Verification items for the finished model (mm, model axes). Face numbers are marked on the shaded views. A direction names the side the tool comes from. Coordinates: 2 decimals unless noted, no trailing zeros. Order: outer loops, then holes, each group sorted by start corner. A loop starts at its lowest first (then second) coordinate and runs counter-clockwise, first axis right, second up. Notation, with made-up numbers: (-22, 88) -> (-14, 88) arc R24 cw to (-14, 120) -> close; hole circle Ø4 at (4.25, 1.5). An arc over 180 degrees is marked (long way). Answer as CSV lines item,"result".
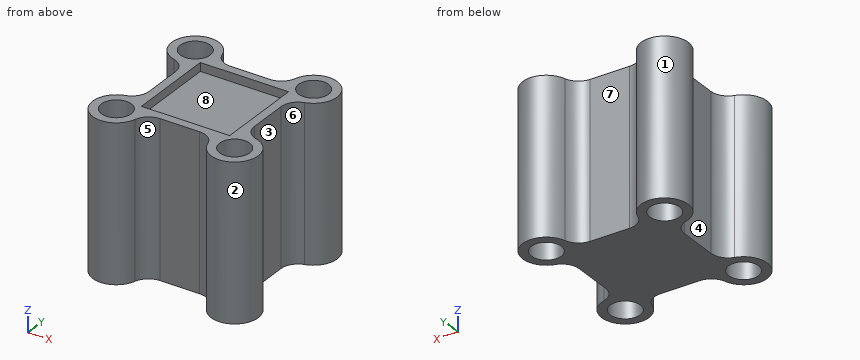
Autodesk Inventor part; units mm, degrees
ref_plane "YZ Plane" through (0, 0, 0) normal (1, 0, 0) x (0, 1, 0)
ref_plane "XZ Plane" through (0, 0, 0) normal (0, 1, 0) x (-1, 0, 0)
ref_plane "XY Plane" through (0, 0, 0) normal (0, 0, 1) x (1, 0, 0)
sketch "Sketch1" plane through (0, 0, 0) normal (0, 0, 1) x (1, 0, 0)
  line L0 (6.15, -6.15) -> (-6.15, -6.15)
  line L1 (-6.15, -6.15) -> (-6.15, 6.15)
  line L2 (-6.15, 6.15) -> (6.15, 6.15)
  line L3 (6.15, 6.15) -> (6.15, -6.15)
  line L4 (6.15, -6.15) -> (-6.15, 6.15) construction
  line L5 (-6.15, -6.15) -> (6.15, 6.15) construction
  line L6 (5.15, -5.15) -> (-5.15, -5.15)
  line L7 (-5.15, -5.15) -> (-5.15, 5.15)
  line L8 (-5.15, 5.15) -> (5.15, 5.15)
  line L9 (5.15, 5.15) -> (5.15, -5.15)
  line L10 (5.15, -5.15) -> (-5.15, 5.15) construction
  line L11 (-5.15, -5.15) -> (5.15, 5.15) construction
  point P0 (0, 0)
  dimension "d0" = 12.3
  dimension "d1" = 12.3
  dimension "d2" = 10.3
extrude "Extrusion1" add sketch "Sketch1" along normal blind 17.1 contours L6 L7 L8 L9
extrude "Extrusion2" add sketch "Sketch1" along normal blind 18.1
sketch "Sketch2" plane through (0, 0, 0) normal (0, 0, 1) x (1, 0, 0)
  line L0 (-6.15, 6.15) -> (-6.15, -6.15) construction
  line L1 (-6.15, 0) -> (6.15, 0)
  line L2 (6.15, -6.15) -> (6.15, 6.15) construction
  line L3 (6.15, 6.15) -> (-6.15, 6.15) construction
  line L4 (0, 6.15) -> (0, -6.15)
  line L5 (-6.15, -6.15) -> (6.15, -6.15) construction
  point P0 (0, 0)
sketch "Sketch3" plane through (0, 0, 0) normal (0, 0, 1) x (1, 0, 0)
  circle A0 centre (-6.9, 6.9) radius 1.75
  line L0 (-11.15, -11.15) -> (11.15, -11.15) construction
  line L1 (11.15, -11.15) -> (11.15, 11.15) construction
  line L2 (11.15, 11.15) -> (-11.15, 11.15) construction
  line L3 (-11.15, 11.15) -> (-11.15, -11.15) construction
  line L4 (-11.15, -11.15) -> (11.15, 11.15) construction
  line L5 (11.15, -11.15) -> (-11.15, 11.15) construction
  line L6 (-6.15, 6.15) -> (-6.15, -6.15)
  line L7 (6.15, 6.15) -> (-6.15, 6.15)
  line L8 (-5.15, 5.15) -> (5.15, 5.15)
  circle A1 centre (6.9, 6.9) radius 1.75
  circle A2 centre (-6.9, -6.9) radius 1.75
  circle A3 centre (6.9, -6.9) radius 1.75
  line L9 (5.15, -5.15) -> (-5.15, -5.15)
  circle A4 centre (-6.9, 6.9) radius 2.75
  circle A5 centre (6.9, 6.9) radius 2.75
  circle A6 centre (6.9, -6.9) radius 2.75
  circle A7 centre (-6.9, -6.9) radius 2.75
  line L10 (5.15, 5.15) -> (-5.15, 5.15)
  line L11 (-5.15, 5.15) -> (-5.15, -5.15)
  line L12 (-5.15, -5.15) -> (5.15, -5.15)
  line L13 (5.15, -5.15) -> (5.15, 5.15)
  point P0 (0, 0)
  point P1 (0, 0)
  point P2 (-4.2542, 6.15)
  point P3 (-6.15, 4.2542)
  point P4 (-5.3189, 6.15)
  point P5 (-6.15, 5.3189)
  point P6 (-4.7787, -5.15)
  point P7 (-5.15, -4.7787)
  point P8 (5.15, -4.7787)
  point P9 (4.7787, -5.15)
  point P10 (-5.15, 4.7787)
  point P11 (-4.7787, 5.15)
  point P12 (4.7787, 5.15)
  point P13 (5.15, 5.15)
  point P14 (5.15, 4.7787)
  dimension "d19" = 3.5
  dimension "d20" = 5
  dimension "d21" = 5
  dimension "d22" = 3.5
  dimension "d23" = 3.5
  dimension "d24" = 3.5
  dimension "d25" = 5.5
  dimension "d26" = 5.5
  dimension "d27" = 5.5
  dimension "d28" = 5.5
extrude "Extrusion4" add sketch "Sketch3" along normal up to surface (18.1 mm away) contours A0 L7 L6 | A0 L6 A4 L7 | L6 L7 A0 | A0 L7 A4 L8 L11 L6 | A2 | A7 L11 L9 | A1 | A5 L13 L8 | L9 L13 A6 | A3 picked at (-4.5292, -7.2681) picked at (5.5596, 5.0279) picked at (4.9749, -5.6466)
extrude "Extrusion5" cut sketch "Sketch3" along normal up to next contours A0 L7 L6 | L6 L7 A0 | A2 | A1 | A3
fillet "Fillet1" radius 2 8 edges at (-4.2542, -6.15, 9.05) (-6.15, -4.2542, 9.05) (-6.15, 4.2542, 9.05) (-4.2542, 6.15, 9.05) (4.2542, 6.15, 9.05) (6.15, 4.2542, 9.05) (6.15, -4.2542, 9.05) (4.2542, -6.15, 9.05)
properties part number "base_cube"
Item 1: Section check B-B, the plane x = 7.25. Record the boundary of the cut face in (y, z), plus the area to 3 significant figures.
Answer list:
outline,"(-9.63, 0) -> (-8.61, 0) -> (-8.61, 18.1) -> (-9.63, 18.1) -> close; (-5.19, 0) -> (-4.1, 0) -> (-4.1, 18.1) -> (-5.19, 18.1) -> close; (4.1, 0) -> (5.19, 0) -> (5.19, 18.1) -> (4.1, 18.1) -> close; (8.61, 0) -> (9.63, 0) -> (9.63, 18.1) -> (8.61, 18.1) -> close"
area,"75.8 mm2"
Item 2: Section check C-C, the plane y = -6.9. Record the boundary of the cut face in (x, z), plus the area to 3 significant figures.
Answer list:
outline,"(-9.65, 0) -> (-8.65, 0) -> (-8.65, 18.1) -> (-9.65, 18.1) -> close; (-5.15, 0) -> (-3.88, 0) -> (-3.88, 18.1) -> (-5.15, 18.1) -> close; (3.88, 0) -> (5.15, 0) -> (5.15, 18.1) -> (3.88, 18.1) -> close; (8.65, 0) -> (9.65, 0) -> (9.65, 18.1) -> (8.65, 18.1) -> close"
area,"82.2 mm2"
Item 3: Depth check by flat-ended pin: pin 1 Ø1.1 at (x, z) = (0, 17.5) entering from -Y; pin 2 Ø0.8 at (y, z) = (0.5, 18) entering from -X; pin 3 Ø5 at (x, z) = (1, 12.5) entering from +Y. Enter the tip coordinate at first touch or a pass-through.
Answer list:
pin 1,"y = -6.15"
pin 2,"x = -6.15"
pin 3,"y = 6.54"
Item 4: Thickness scan on line 1 (X direction, y = 6.9, z = 10); line 2 (X direction, y = -5.75, z = 0.75). Record the ranges inside material, lowest first.
Answer list:
line 1,"-9.65 to -8.65, -5.15 to -3.88, 3.88 to 5.15, 8.65 to 9.65"
line 2,"-9.4 to -8.22, -5.58 to 5.58, 8.22 to 9.4"
Item 5: Release check for a two-part mould opening along X. For the marked faces 1, 2, 3 and 4 record: +X half, -X half, draft (parallel to the pull), parting line (faces both ways), or undercut.
Answer list:
face 1,"undercut"
face 2,"undercut"
face 3,"+X half"
face 4,"-X half"
Item 6: Section check A-A, the plane z = 9.5. Record the boundary of the cut face in (x, y).
Answer list:
outline,"(-7.62, -4.25) arc R2.75 ccw (long way) to (-4.25, -7.62) arc R2 cw to (-2.32, -6.15) -> (2.32, -6.15) arc R2 cw to (4.25, -7.62) arc R2.75 ccw (long way) to (7.62, -4.25) arc R2 cw to (6.15, -2.32) -> (6.15, 2.32) arc R2 cw to (7.62, 4.25) arc R2.75 ccw (long way) to (4.25, 7.62) arc R2 cw to (2.32, 6.15) -> (-2.32, 6.15) arc R2 cw to (-4.25, 7.62) arc R2.75 ccw (long way) to (-7.62, 4.25) arc R2 cw to (-6.15, 2.32) -> (-6.15, -2.32) arc R2 cw to start; hole circle Ø3.5 at (-6.9, -6.9); hole circle Ø3.5 at (-6.9, 6.9); hole circle Ø3.5 at (6.9, -6.9); hole circle Ø3.5 at (6.9, 6.9)"
Item 7: Section check D-D, the plane x = -1. Record the boundary of the cut face in (y, z).
Answer list:
outline,"(-6.15, 0) -> (6.15, 0) -> (6.15, 18.1) -> (5.15, 18.1) -> (5.15, 17.1) -> (-5.15, 17.1) -> (-5.15, 18.1) -> (-6.15, 18.1) -> close"
Item 8: Tool access check on the marked faces 5, 6, 7 and 8. Record the directions out of +Z, -Z, +X, -X, +Y, -Y that give a thin tool (end or side, any length) a straight path to the whole face; none if there is none.
Answer list:
face 5,"+Z, -Z, -Y"
face 6,"+Z, -Z, +X"
face 7,"+Z, -Z, +Y"
face 8,"+Z"
